from build123d import *

# Parameters (mm, degrees)
SKETCH1_R           = 47.625
BOSS_EXTRUDE1_DEPTH = 12.7
SKETCH6_R           = 1.7526
CUT_EXTRUDE3_DEPTH  = 19.05
CIRPATTERN4_COUNT   = 4
SKETCH7_R           = 3.175
CUT_EXTRUDE6_DEPTH  = 69.538830402
SKETCH8_R           = 4.7625
CUT_EXTRUDE7_DEPTH  = 69.538830402
SKETCH11_R          = 2.38125
CUT_EXTRUDE8_DEPTH  = 69.538830402


with BuildPart() as part:
    # Sketch1 → Boss-Extrude1 (new body)
    with BuildSketch(Plane(origin=(0, 0, 0), x_dir=(1, 0, 0), z_dir=(0, 1, 0))):
        with Locations(Location((0, 0, 0), (0, 0, 270))):
            Circle(SKETCH1_R)
    extrude(amount=BOSS_EXTRUDE1_DEPTH)

    # Sketch6 → Cut-Extrude3 (cut)
    with BuildSketch(Plane(origin=(0, 0, -47.625), x_dir=(0, -1, 0), z_dir=(0, 0, -1))):
        with Locations(Location((-6.35, 0, 0), (0, 0, 90))):
            Circle(SKETCH6_R)
    cut_extrude3 = extrude(amount=-CUT_EXTRUDE3_DEPTH, mode=Mode.SUBTRACT)

    # CirPattern4: Cut-Extrude3 ×4 about axis
    cirpattern4_axis = Axis((0, 0, 0), (0, 1, 0))
    for i in range(1, CIRPATTERN4_COUNT):
        add(cut_extrude3.rotate(cirpattern4_axis, i * 360 / CIRPATTERN4_COUNT), mode=Mode.SUBTRACT)

    # Sketch7 → Cut-Extrude6 (cut, through all)
    with BuildSketch(Plane(origin=(0, 0, 0), x_dir=(1, 0, 0), z_dir=(0, 1, 0))):
        with Locations(Location((-26.19375, 0, 0), (0, 0, 270))):
            Circle(SKETCH7_R)
        with Locations(Location((26.19375, 0, 0), (0, 0, 270))):
            Circle(SKETCH7_R)
        with Locations(Location((0, 26.19375, 0), (0, 0, 270))):
            Circle(SKETCH7_R)
        with Locations(Location((0, -26.19375, 0), (0, 0, 270))):
            Circle(SKETCH7_R)
    extrude(amount=CUT_EXTRUDE6_DEPTH, mode=Mode.SUBTRACT)

    # Sketch8 → Cut-Extrude7 (cut, through all)
    with BuildSketch(Plane(origin=(0, 12.7, 0), x_dir=(1, 0, 0), z_dir=(0, 1, 0))):
        with Locations(Location((0, 0, 0), (0, 0, 270))):
            Circle(SKETCH8_R)
    extrude(amount=-CUT_EXTRUDE7_DEPTH, mode=Mode.SUBTRACT)

    # Sketch11 → Cut-Extrude8 (cut, through all)
    with BuildSketch(Plane(origin=(0, 12.7, 0), x_dir=(1, 0, 0), z_dir=(0, 1, 0))):
        with Locations(Location((31.589006405, 31.589006405, 0), (0, 0, 270))):
            Circle(SKETCH11_R)
        with Locations(Location((40.488032715, 18.879879719, 0), (0, 0, 270))):
            Circle(SKETCH11_R)
        with Locations(Location((18.879879719, 40.488032715, 0), (0, 0, 270))):
            Circle(SKETCH11_R)
        with Locations(Location((40.488032715, -18.879879719, 0), (0, 0, 270))):
            Circle(SKETCH11_R)
    extrude(amount=-CUT_EXTRUDE8_DEPTH, mode=Mode.SUBTRACT)


solid = part.part
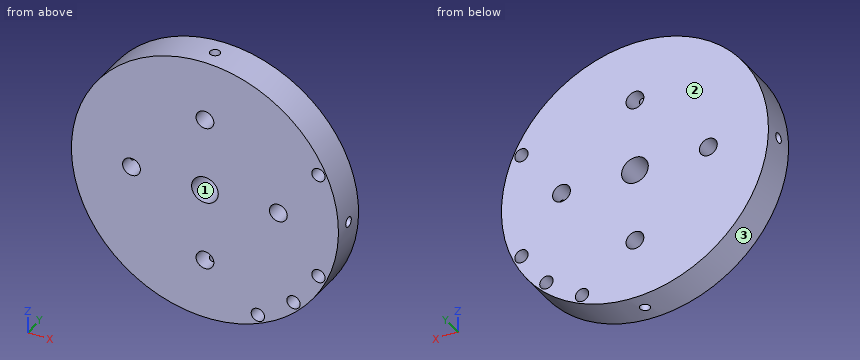
The model under review builds one solid part; all positions refer to its coordinate system, in mm. Face numbers are marked on the shaded views. Coordinates: 2 decimals unless noted, no trailing zeros. Write each loop counter-clockwise with the first axis right and the second up, starting at its lowest first coordinate (ties: lowest second). Pieces come first, ordered by that corner, then holes. Notation, with made-up numbers: M 19.25,53.5 L 70.25,53.5 A20 cw 70.25,58.5 Z; hole C 88.5,-5.5 d4. An arc over 180 degrees is marked long. Put each result on its own line as item: value.
1) Draft analysis for pull direction Z (two halves, no side actions). For the marked faces 1, 2 and 3, state which applies: released by +Z, released by -Z, zero draft, split by the parting line, or undercut.
Computed:
face 1: undercut
face 2: zero draft
face 3: split by the parting line
2) Add section A-A on x = 0. Give the boundary of the cut face in (y, z) (1 decimal), then the cut area to 3 significant figures.
Computed:
outline: M 0,-47.6 L 4.6,-47.6 L 4.6,-29.4 L 0,-29.4 Z; M 0,-23 L 12.7,-23 L 12.7,-4.8 L 0,-4.8 Z; M 0,4.8 L 12.7,4.8 L 12.7,23 L 0,23 Z; M 0,29.4 L 4.6,29.4 L 4.6,47.6 L 0,47.6 Z; M 8.1,-47.6 L 12.7,-47.6 L 12.7,-29.4 L 8.1,-29.4 Z; M 8.1,29.4 L 12.7,29.4 L 12.7,47.6 L 8.1,47.6 Z
area: 799 mm2
3) Clearance check with flat-ended pins moving along their axes: pin 1 Ø4 at (x, y) = (0, 6.35) entering from +Z (3 decimals); pin 2 Ø5 at (x, y) = (-10, 7) entering from -Z; pin 3 Ø2 at (x, y) = (21.5, 5) entering from -Z; pin 4 Ø1 at (x, y) = (32, 5.5) entering from +Z. State where each tip first meets the part, or that it passes through.
Computed:
pin 1: stops at z = 47.625
pin 2: stops at z = -47.03
pin 3: stops at z = -42.99
pin 4: stops at z = 35.72
4) Add section C-C on y = 6.35. State how many separate pieces and enclosed holes the cut face has, then the cut area to 3 significant figures.
Computed:
separate pieces: 1
enclosed holes: 5
area: 6,600 mm2
5) Add section D-D on z = 25. Give the boundary of the cut face in (x, y), then the cut area to 3 significant figures.
Computed:
outline: M -40.54,0 L -2.94,0 L -2.94,12.7 L -40.54,12.7 Z; M 2.94,0 L 40.54,0 L 40.54,12.7 L 2.94,12.7 Z
area: 955 mm2
6) Wall thickness on probe 1 along X at (y, z) = (9.5, 1.5); probe 2 along X at (y, z) = (4.75, -1); probe 3 along Z at (x, y) = (-31, 5.25): over which ranges is each line inside the solid? List them lowest first. Write a range as [from, to].
Computed:
probe 1: x = [-47.6, -28.99], [-23.4, -4.52], [4.52, 23.4], [28.99, 47.6]
probe 2: x = [-47.61, -29.21], [-23.18, -4.66], [4.66, 23.18], [29.21, 47.61]
probe 3: z = [-36.15, -1.36], [1.36, 36.15]
7) Add section B-B on z = 0. Give the boundary of the cut face in (x, y) (1 decimal), then the cut area to 3 significant figures.
Computed:
outline: M -47.6,0 L -29.4,0 L -29.4,4.6 L -47.6,4.6 Z; M -47.6,8.1 L -29.4,8.1 L -29.4,12.7 L -47.6,12.7 Z; M -23,0 L -4.8,0 L -4.8,12.7 L -23,12.7 Z; M 4.8,0 L 23,0 L 23,12.7 L 4.8,12.7 Z; M 29.4,0 L 47.6,0 L 47.6,4.6 L 29.4,4.6 Z; M 29.4,8.1 L 47.6,8.1 L 47.6,12.7 L 29.4,12.7 Z
area: 799 mm2
